from build123d import *

# Parameters (mm, degrees)
SKETCH1_R           = 21
SKETCH1_R_2         = 1.25
SKETCH1_R_3         = 11
BOSS_EXTRUDE1_DEPTH = 3
SKETCH1_3_R         = 3
SKETCH1_3_R_2       = 1.25
BOSS_EXTRUDE2_DEPTH = 3
BOSS_EXTRUDE3_DEPTH = 20
SKETCH5_R           = 21.5
SKETCH5_R_2         = 11
SKETCH5_R_3         = 1.25
BOSS_EXTRUDE4_DEPTH = 6
BOSS_EXTRUDE5_DEPTH = 3


with BuildPart() as part:
    # Sketch1 → Boss-Extrude1 (new body)
    with BuildSketch(Plane.XY):
        Circle(SKETCH1_R)
        with Locations((-13.081475452, 13.081475452)):
            Circle(SKETCH1_R_2, mode=Mode.SUBTRACT)
        with Locations((13.081475452, 13.081475452)):
            Circle(SKETCH1_R_2, mode=Mode.SUBTRACT)
        with Locations((13.081475452, -13.081475452)):
            Circle(SKETCH1_R_2, mode=Mode.SUBTRACT)
        with Locations((-13.081475452, -13.081475452)):
            Circle(SKETCH1_R_2, mode=Mode.SUBTRACT)
        Circle(SKETCH1_R_3, mode=Mode.SUBTRACT)
    extrude(amount=BOSS_EXTRUDE1_DEPTH)

    # Sketch1_3 → Boss-Extrude2 (add)
    with BuildSketch(Plane.XY):
        with BuildLine():
            ThreePointArc((0, 16), (-3.121445152, 15.692564486), (-6.122934918, 14.78207252))
            Line((-6.122934918, 14.78207252), (-8.03635208, 19.401470183))
            ThreePointArc((-8.03635208, 19.401470183), (-14.849242405, 14.849242405), (-19.401470183, 8.03635208))
            Line((-19.401470183, 8.03635208), (-14.78207252, 6.122934918))
            ThreePointArc((-14.78207252, 6.122934918), (-16, 0), (-14.78207252, -6.122934918))
            Line((-14.78207252, -6.122934918), (-19.401470183, -8.03635208))
            ThreePointArc((-19.401470183, -8.03635208), (-14.849242405, -14.849242405), (-8.03635208, -19.401470183))
            Line((-8.03635208, -19.401470183), (-6.122934918, -14.78207252))
            ThreePointArc((-6.122934918, -14.78207252), (0, -16), (6.122934918, -14.78207252))
            Line((6.122934918, -14.78207252), (8.03635208, -19.401470183))
            ThreePointArc((8.03635208, -19.401470183), (14.849242405, -14.849242405), (19.401470183, -8.03635208))
            Line((19.401470183, -8.03635208), (14.78207252, -6.122934918))
            ThreePointArc((14.78207252, -6.122934918), (16, 0), (14.78207252, 6.122934918))
            Line((14.78207252, 6.122934918), (19.401470183, 8.03635208))
            ThreePointArc((19.401470183, 8.03635208), (14.849242405, 14.849242405), (8.03635208, 19.401470183))
            Line((8.03635208, 19.401470183), (6.122934918, 14.78207252))
            ThreePointArc((6.122934918, 14.78207252), (3.121445152, 15.692564486), (0, 16))
        make_face()
        Circle(SKETCH1_3_R, mode=Mode.SUBTRACT)
        with Locations((-13.081475452, -13.081475452)):
            Circle(SKETCH1_3_R_2, mode=Mode.SUBTRACT)
        with Locations((13.081475452, -13.081475452)):
            Circle(SKETCH1_3_R_2, mode=Mode.SUBTRACT)
        with Locations((-13.081475452, 13.081475452)):
            Circle(SKETCH1_3_R_2, mode=Mode.SUBTRACT)
        with Locations((13.081475452, 13.081475452)):
            Circle(SKETCH1_3_R_2, mode=Mode.SUBTRACT)
    extrude(amount=-BOSS_EXTRUDE2_DEPTH)

    # Sketch2 → Boss-Extrude3 (add)
    with BuildSketch(Plane.XY.offset(3)):
        with BuildLine():
            ThreePointArc((8.03635208, 19.401470183), (0, 21), (-8.03635208, 19.401470183))
            Line((-8.03635208, 19.401470183), (-4.209517756, 10.162674858))
            ThreePointArc((-4.209517756, 10.162674858), (0, 11), (4.209517756, 10.162674858))
            Line((4.209517756, 10.162674858), (8.03635208, 19.401470183))
        make_face()
        with BuildLine():
            Line((-10.162674858, 4.209517756), (-19.401470183, 8.03635208))
            ThreePointArc((-19.401470183, 8.03635208), (-21, 0), (-19.401470183, -8.03635208))
            Line((-19.401470183, -8.03635208), (-10.162674858, -4.209517756))
            ThreePointArc((-10.162674858, -4.209517756), (-11, 0), (-10.162674858, 4.209517756))
        make_face()
        with BuildLine():
            Line((-4.209517756, -10.162674858), (-8.03635208, -19.401470183))
            ThreePointArc((-8.03635208, -19.401470183), (0, -21), (8.03635208, -19.401470183))
            Line((8.03635208, -19.401470183), (4.209517756, -10.162674858))
            ThreePointArc((4.209517756, -10.162674858), (0, -11), (-4.209517756, -10.162674858))
        make_face()
        with BuildLine():
            ThreePointArc((21, 0), (20.596490888, 4.096896762), (19.401470183, 8.03635208))
            Line((19.401470183, 8.03635208), (10.162674858, 4.209517756))
            ThreePointArc((10.162674858, 4.209517756), (10.788638084, 2.145993542), (11, 0))
            ThreePointArc((11, 0), (10.788638084, -2.145993542), (10.162674858, -4.209517756))
            Line((10.162674858, -4.209517756), (19.401470183, -8.03635208))
            ThreePointArc((19.401470183, -8.03635208), (20.596490888, -4.096896762), (21, 0))
        make_face()
    extrude(amount=BOSS_EXTRUDE3_DEPTH)

    # Sketch5 → Boss-Extrude4 (add)
    with BuildSketch(Plane.XY.offset(23)):
        Circle(SKETCH5_R)
        Circle(SKETCH5_R_2, mode=Mode.SUBTRACT)
        with Locations((-13.435028843, 13.435028843)):
            Circle(SKETCH5_R_3, mode=Mode.SUBTRACT)
        with Locations((13.435028843, 13.435028843)):
            Circle(SKETCH5_R_3, mode=Mode.SUBTRACT)
        with Locations((13.435028843, -13.435028843)):
            Circle(SKETCH5_R_3, mode=Mode.SUBTRACT)
        with Locations((-13.435028843, -13.435028843)):
            Circle(SKETCH5_R_3, mode=Mode.SUBTRACT)
    extrude(amount=BOSS_EXTRUDE4_DEPTH)

    # Sketch6 → Boss-Extrude5 (add)
    with BuildSketch(Plane.XY.offset(29)):
        with BuildLine():
            ThreePointArc((-15.244012286, -6.314276634), (-16.5, 0), (-15.244012286, 6.314276634))
            Line((-15.244012286, 6.314276634), (-19.863409949, 8.227693796))
            ThreePointArc((-19.863409949, 8.227693796), (-21.5, 0), (-19.863409949, -8.227693796))
            Line((-19.863409949, -8.227693796), (-15.244012286, -6.314276634))
        make_face()
        with BuildLine():
            Line((-8.227693796, 19.863409949), (-6.314276634, 15.244012286))
            ThreePointArc((-6.314276634, 15.244012286), (0, 16.5), (6.314276634, 15.244012286))
            Line((6.314276634, 15.244012286), (8.227693796, 19.863409949))
            ThreePointArc((8.227693796, 19.863409949), (0, 21.5), (-8.227693796, 19.863409949))
        make_face()
        with BuildLine():
            ThreePointArc((6.314276634, -15.244012286), (0, -16.5), (-6.314276634, -15.244012286))
            Line((-6.314276634, -15.244012286), (-8.227693796, -19.863409949))
            ThreePointArc((-8.227693796, -19.863409949), (0, -21.5), (8.227693796, -19.863409949))
            Line((8.227693796, -19.863409949), (6.314276634, -15.244012286))
        make_face()
        with BuildLine():
            Line((19.863409949, 8.227693796), (15.244012286, 6.314276634))
            ThreePointArc((15.244012286, 6.314276634), (16.5, 0), (15.244012286, -6.314276634))
            Line((15.244012286, -6.314276634), (19.863409949, -8.227693796))
            ThreePointArc((19.863409949, -8.227693796), (21.5, 0), (19.863409949, 8.227693796))
        make_face()
    extrude(amount=BOSS_EXTRUDE5_DEPTH)


solid = part.part
Can you work these out from the model? Positions are in its coordinate system, mm. A direction names the side the tool comes from. Round coordinates to 2 decimals unless told otherwise and drop trailing zeros. Loops run counter-clockwise (first coordinate to the right, second up) from the corner with the lowest first, then second, coordinate; pieces in that order, holes last. Notation, with made-up numbers: (13.5, -17.5) - (44.5, -17.5) arc R17 ccw to (44.5, 0.5) - close; hole circle Ø7 at (39.5, 3). An arc over 180 degrees is marked (long way). Use CSV: the item, a comma, the result in double quotes. Start each with the question number.
1) We'd pull the mould along X, two halves only. Please class faces 1 (the flat face through (6.15, -14.85, 12.86)), 2 (the flat face through (-18, 0, 32)), 3 (the flat face through (7.066, -17.059, -1.479)): released by +X, released by -X, zero draft, split by the parting line, or undercut.
2) Please list where these lines run through material, in increasing order: probe 1 along Z at (x, y) = (13, -15.5); probe 2 along Y at (x, z) = (0, 1.9); probe 3 along Y at (x, z) = (0, -1.95). Write a range as [from, to].
3) If we section it at B-B on x = -17.5: Write out the boundary of the cut face in (y, z), plus the area to 3 significant figures.
4) If we section it at C-C on y = 1: Write out the boundary of the cut face in (x, z).
5) For faces 4 (the flat face through (-8, -8, 23)), 5 (the flat face through (7.09, 17.12, -1.48)), 6 (the cylindrical face through (12.92, -11.84, -0.04)), 7 (the flat face through (-9, -9, 29)), 8 (the cylindrical face through (-16, 0, -1)), which set-ups out of +Z, -Z, +X, -X, +Y, -Y let a thin tool reach every point of the face, with its end or its side?
6) For pin 1 Ø17.5 at (x, y) = (0.5, 1.5) entering from +Z; pin 2 Ø2 at (x, z) = (15, 2.5) entering from -Y; pin 3 Ø3 at (x, y) = (-13.44, 13.44) entering from +Z; pin 4 Ø4 at (x, y) = (-13.08, -13.08) entering from -Z, each with a flat end and sliding along its axis, tell me the tip position at first contact or that it passes through.
7) If we section it at A-A on z = 10.5: Write out the boundary of the cut face in (x, y), plus the area to 3 significant figures.
8) If we section it at D-D on z = -1: Write out the boundary of the cut face in (x, y).
Geometry results:
1,face 1,"released by +X"
1,face 2,"zero draft"
1,face 3,"undercut"
2,probe 1,"z = [-3, 3], [23, 29]"
2,probe 2,"y = [-21, -11], [11, 21]"
2,probe 3,"y = [-16, -3], [3, 16]"
3,outline,"(-12.49, 23) - (-7.25, 23) - (-7.25, 3) - (-11.61, 3) - (-11.61, -3) - (-7.25, -3) - (-7.25, 0) - (7.25, 0) - (7.25, -3) - (11.61, -3) - (11.61, 3) - (7.25, 3) - (7.25, 23) - (12.49, 23) - (12.49, 29) - (7.25, 29) - (7.25, 32) - (-7.25, 32) - (-7.25, 29) - (-12.49, 29) - close"
3,area,"579 mm2"
4,outline,"(-21.48, 23) - (-20.98, 23) - (-20.98, 0) - (-15.97, 0) - (-15.97, -3) - (-2.83, -3) - (-2.83, 0) - (-10.95, 0) - (-10.95, 29) - (-16.47, 29) - (-16.47, 32) - (-21.48, 32) - close; (2.83, -3) - (15.97, -3) - (15.97, 0) - (20.98, 0) - (20.98, 23) - (21.48, 23) - (21.48, 32) - (16.47, 32) - (16.47, 29) - (10.95, 29) - (10.95, 0) - (2.83, 0) - close"
5,face 4,"none"
5,face 5,"-Z, +Y"
5,face 6,"-Z"
5,face 7,"+Z"
5,face 8,"-Z, -X"
6,pin 1,"stops at z = 0"
6,pin 2,"stops at y = -15.65"
6,pin 3,"stops at z = 29"
6,pin 4,"stops at z = -3"
7,outline,"(-19.4, -8.04) - (-10.16, -4.21) arc R11 cw to (-10.16, 4.21) - (-19.4, 8.04) arc R21 ccw to start; (-8.04, -19.4) arc R21 ccw to (8.04, -19.4) - (4.21, -10.16) arc R11 cw to (-4.21, -10.16) - close; (-8.04, 19.4) - (-4.21, 10.16) arc R11 cw to (4.21, 10.16) - (8.04, 19.4) arc R21 ccw to start; (10.16, -4.21) - (19.4, -8.04) arc R21 ccw to (19.4, 8.04) - (10.16, 4.21) arc R11 cw to start"
7,area,"503 mm2"
8,outline,"(-19.4, -8.04) arc R21 ccw to (-8.04, -19.4) - (-6.12, -14.78) arc R16 ccw to (6.12, -14.78) - (8.04, -19.4) arc R21 ccw to (19.4, -8.04) - (14.78, -6.12) arc R16 ccw to (14.78, 6.12) - (19.4, 8.04) arc R21 ccw to (8.04, 19.4) - (6.12, 14.78) arc R16 ccw to (-6.12, 14.78) - (-8.04, 19.4) arc R21 ccw to (-19.4, 8.04) - (-14.78, 6.12) arc R16 ccw to (-14.78, -6.12) - close; hole circle Ø2.5 at (-13.08, -13.08); hole circle Ø2.5 at (-13.08, 13.08); hole circle Ø6 at (0, 0); hole circle Ø2.5 at (13.08, -13.08); hole circle Ø2.5 at (13.08, 13.08)"
